from build123d import *

# Parameters (mm, degrees)
SKETCH1_W           = 31.5
SKETCH1_H           = 38
BOSS_EXTRUDE1_DEPTH = 5
SKETCH3_W           = 64
SKETCH3_H           = 38
BOSS_EXTRUDE3_DEPTH = 5
SKETCH7_R           = 1.05
CUT_EXTRUDE3_DEPTH  = 5
SKETCH8_W           = 10
SKETCH8_H           = 38
CUT_EXTRUDE4_DEPTH  = 10
FILLET1_R           = 5
SKETCH9_R           = 2
CUT_EXTRUDE5_DEPTH  = 1.5
SKETCH11_R          = 2
CUT_EXTRUDE7_DEPTH  = 1.5
CUT_EXTRUDE8_DEPTH  = 39


with BuildPart() as part:
    # Sketch1 → Boss-Extrude1 (new body)
    with BuildSketch(Plane(origin=(0, 0, 0), x_dir=(0, 0, -1), z_dir=(1, 0, 0))):
        with Locations((3.25, 0)):
            Rectangle(SKETCH1_W, SKETCH1_H)
        with BuildLine():
            ThreePointArc((1.05, 8), (0, 9.05), (-1.05, 8))
            ThreePointArc((-1.05, 8), (0, 6.95), (1.05, 8))
        make_face(mode=Mode.SUBTRACT)
        with BuildLine():
            ThreePointArc((6.95, 0), (8, -1.05), (9.05, 0))
            ThreePointArc((9.05, 0), (8, 1.05), (6.95, 0))
        make_face(mode=Mode.SUBTRACT)
        with BuildLine():
            ThreePointArc((-1.05, -8), (0, -9.05), (1.05, -8))
            ThreePointArc((1.05, -8), (0, -6.95), (-1.05, -8))
        make_face(mode=Mode.SUBTRACT)
        with BuildLine():
            ThreePointArc((-9.05, 0), (-8, -1.05), (-6.95, 0))
            ThreePointArc((-6.95, 0), (-8, 1.05), (-9.05, 0))
        make_face(mode=Mode.SUBTRACT)
    extrude(amount=BOSS_EXTRUDE1_DEPTH)

    # Sketch3 → Boss-Extrude3 (add)
    with BuildSketch(Plane(origin=(0, 0, -19), x_dir=(-1, 0, 0), z_dir=(0, 0, -1))):
        with Locations((-32, 0)):
            Rectangle(SKETCH3_W, SKETCH3_H)
    extrude(amount=BOSS_EXTRUDE3_DEPTH)

    # Sketch7 → Cut-Extrude3 (cut)
    with BuildSketch(Plane.XY.offset(-19)):
        with Locations((33.5, 8)):
            Circle(SKETCH7_R)
        with Locations((33.5, -8)):
            Circle(SKETCH7_R)
        with BuildLine():
            ThreePointArc((41.5, -6.95), (40.45, -8), (41.5, -9.05))
            ThreePointArc((41.5, -9.05), (42.55, -8), (41.5, -6.95))
        make_face()
        with BuildLine():
            ThreePointArc((41.5, 9.05), (40.45, 8), (41.5, 6.95))
            ThreePointArc((41.5, 6.95), (42.55, 8), (41.5, 9.05))
        make_face()
    extrude(amount=-CUT_EXTRUDE3_DEPTH, mode=Mode.SUBTRACT)

    # Sketch8 → Cut-Extrude4 (cut)
    with BuildSketch(Plane(origin=(0, 0, -24), x_dir=(-1, 0, 0), z_dir=(0, 0, -1))):
        with Locations((-59, 0)):
            Rectangle(SKETCH8_W, SKETCH8_H)
    extrude(amount=-CUT_EXTRUDE4_DEPTH, mode=Mode.SUBTRACT)

    # Fillet1
    fillet1_edges = [part.edges().sort_by_distance(p)[0] for p in [
        (0, 0, -24),
        (5, 0, -19),
    ]]
    fillet(fillet1_edges, radius=FILLET1_R)

    # Sketch9 → Cut-Extrude5 (cut)
    with BuildSketch(Plane(origin=(0, 0, -24), x_dir=(-1, 0, 0), z_dir=(0, 0, -1))):
        with Locations((-41.5, 8)):
            Circle(SKETCH9_R)
        with Locations((-41.5, -8)):
            Circle(SKETCH9_R)
        with Locations((-33.5, 8)):
            Circle(SKETCH9_R)
        with Locations((-33.5, -8)):
            Circle(SKETCH9_R)
    extrude(amount=-CUT_EXTRUDE5_DEPTH, mode=Mode.SUBTRACT)

    # Sketch11 → Cut-Extrude7 (cut)
    with BuildSketch(Plane(origin=(5, 0, 0), x_dir=(0, 0, -1), z_dir=(1, 0, 0))):
        with Locations((0, 8)):
            Circle(SKETCH11_R)
        with Locations((-8, 0)):
            Circle(SKETCH11_R)
        with Locations((0, -8)):
            Circle(SKETCH11_R)
        with Locations((8, 0)):
            Circle(SKETCH11_R)
    extrude(amount=-CUT_EXTRUDE7_DEPTH, mode=Mode.SUBTRACT)

    # Sketch12 → Cut-Extrude8 (cut, through all)
    with BuildSketch(Plane(origin=(0, 19, 0), x_dir=(1, 0, 0), z_dir=(0, 1, 0))):
        Polygon((54, 24), (49, 24), (49, 17.432960287), (56.636110038, 15.929403626), (56.327583627, 23.530489308), align=None)
    extrude(amount=-CUT_EXTRUDE8_DEPTH, mode=Mode.SUBTRACT)


solid = part.part
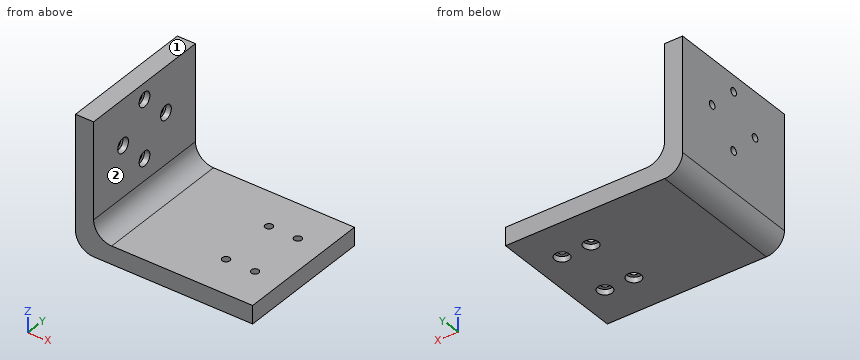
Here's how the part is built. I have some questions about the finished solid (model axes, mm). Face numbers are marked on the shaded views. A direction names the side the tool comes from. Round coordinates to 2 decimals unless told otherwise and drop trailing zeros. Write each loop counter-clockwise with the first axis right and the second up, starting at its lowest first coordinate (ties: lowest second). Pieces come first, ordered by that corner, then holes.
1. Suppose I cut it at D-D (y = 8). State how many separate pieces and enclosed holes the cut face has, and give its area (3 significant figures).
2. Suppose I cut it at A-A (z = 0). List the corners of the cut face in (x, y) for me, and give its area (3 significant figures).
3. Will these pins go through, and if not, where does the flat tip stop? pin 1 Ø2.5 at (x, y) = (41.5, -8) entering from -Z; pin 2 Ø3 at (x, y) = (41.5, 8) entering from +Z; pin 3 Ø1.7 at (y, z) = (8, 0) entering from +X; pin 4 Ø5 at (y, z) = (0, 8) entering from +X.
4. Suppose I cut it at C-C (z = 8). List the corners of the cut face in (x, y) for me.
5. Suppose I cut it at B-B (y = 0). List the corners of the cut face in (x, z) for me, and give its area (3 significant figures).
6. I need wall thicknesses on L1, parallel to Y at x = 3, z = 8; L2, parallel to Y at x = 41, z = -20; L3, parallel to Y at x = 2.2, z = 0. Which ranges of each line are inside material? Lowest first, please.
7. For the marked faces 1 and 2, which set-ups out of +Z, -Z, +X, -X, +Y, -Y let a thin tool reach every point of the face, with its end or its side?
Answer sheet:
1. separate pieces: 4
1. enclosed holes: 0
1. area: 362 mm2
2. outline: (0, -19) - (5, -19) - (5, -10) - (3.5, -10) - (3.5, -9.05) - (0, -9.05) - close; (0, -6.95) - (3.5, -6.95) - (3.5, -6) - (5, -6) - (5, 6) - (3.5, 6) - (3.5, 6.95) - (0, 6.95) - close; (0, 9.05) - (3.5, 9.05) - (3.5, 10) - (5, 10) - (5, 19) - (0, 19) - close
2. area: 163 mm2
3. pin 1: stops at z = -22.5
3. pin 2: stops at z = -19
3. pin 3: passes through
3. pin 4: stops at x = 5
4. outline: (0, -19) - (5, -19) - (5, -2) - (3.5, -2) - (3.5, -1.05) - (0, -1.05) - close; (0, 1.05) - (3.5, 1.05) - (3.5, 2) - (5, 2) - (5, 19) - (0, 19) - close
5. outline: (0, -19) arc R5 ccw to (5, -24) - (49, -24) - (49, -19) - (10, -19) arc R5 cw to (5, -14) - (5, -10) - (3.5, -10) - (3.5, -9.05) - (0, -9.05) - close; (0, -6.95) - (3.5, -6.95) - (3.5, -6) - (5, -6) - (5, 6) - (3.5, 6) - (3.5, 6.95) - (0, 6.95) - close; (0, 9.05) - (3.5, 9.05) - (3.5, 10) - (5, 10) - (5, 12.5) - (0, 12.5) - close
5. area: 376 mm2
6. L1: y = -19 to -1.05, 1.05 to 19
6. L2: y = -19 to -8.92, -7.08 to 7.08, 8.92 to 19
6. L3: y = -19 to -9.05, -6.95 to 6.95, 9.05 to 19
7. face 1: +Z, +X, -X, +Y, -Y
7. face 2: +Z, +X, +Y, -Y
